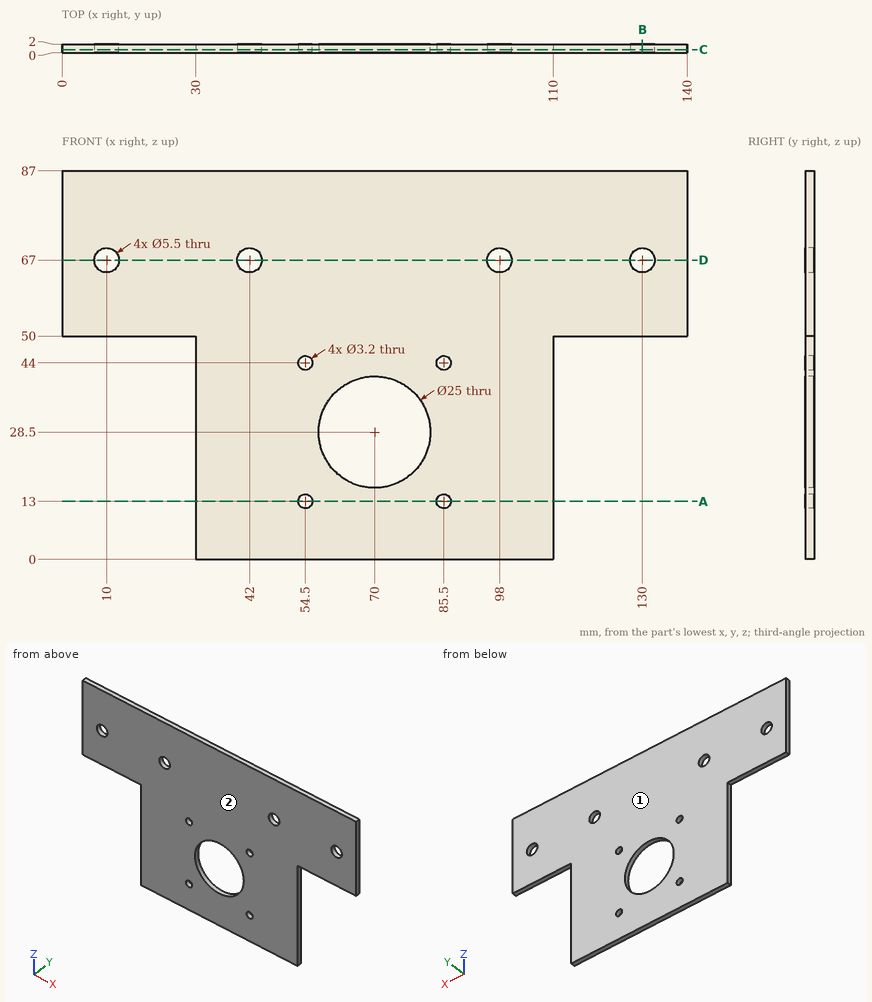
Could you check a few things on this drawing? It's one solid part, dimensions in mm from its lowest x, y, z. Coordinates: 2 decimals unless noted, no trailing zeros. Order: outer loops, then holes, each group sorted by start corner. A loop starts at its lowest first (then second) coordinate and runs counter-clockwise, first axis right, second up. Notation, with made-up numbers: M 5.25,37 L 44.25,37 A16 ccw 44.25,49 Z; hole C 42.25,20 d3. An arc over 180 degrees is marked long. Use one line per item in the form item = value. Start each with the question number.
1. We'd pull the mould along Y, two halves only. Please class the marked faces 1 and 2: +Y half, -Y half, draft (parallel to the pull), parting line (faces both ways), or undercut.
2. For pin 1 (12 mm diameter, centred on x = 124.5, z = 70.5, fed in from -Y); pin 2 (4.5 mm diameter, centred on x = 10, z = 67, fed in from -Y), each with a flat end and sliding along its axis, tell me the tip position at first contact or that it passes through.
3. Suppose I cut it at A-A on z = 13. Write out the boundary of the cut face in (x, y).
4. Please list where these lines run through material, in increasing order: line 1 (Z direction, x = 54.5, y = 1.4); line 2 (X direction, y = 1.55, z = 67); line 3 (Z direction, x = 130, y = 1.2).
5. Suppose I cut it at B-B on x = 130. Write out the boundary of the cut face in (y, z), then the cut area to 3 significant figures.
6. Suppose I cut it at C-C on y = 0.75. Count the separate pieces of the cut face and the enclosed holes in it, then the cut area to 3 significant figures.
7. Suppose I cut it at D-D on z = 67. Write out the boundary of the cut face in (x, y).
Geometry says:
q1.face_1 = +Y half
q1.face_2 = -Y half
q2.pin_1 = 0
q2.pin_2 = through
q3.outline = M 30,0 L 52.9,0 L 52.9,2 L 30,2 Z; M 56.1,0 L 83.9,0 L 83.9,2 L 56.1,2 Z; M 87.1,0 L 110,0 L 110,2 L 87.1,2 Z
q4.line_1 = 0 to 11.4, 14.6 to 42.4, 45.6 to 87
q4.line_2 = 0 to 7.25, 12.75 to 39.25, 44.75 to 95.25, 100.75 to 127.25, 132.75 to 140
q4.line_3 = 50 to 64.25, 69.75 to 87
q5.outline = M 0,50 L 2,50 L 2,64.25 L 0,64.25 Z; M 0,69.75 L 2,69.75 L 2,87 L 0,87 Z
q5.area = 63.0 mm^2
q6.separate_pieces = 1
q6.enclosed_holes = 9
q6.area = 8,560 mm^2
q7.outline = M 0,0 L 7.25,0 L 7.25,2 L 0,2 Z; M 12.75,0 L 39.25,0 L 39.25,2 L 12.75,2 Z; M 44.75,0 L 95.25,0 L 95.25,2 L 44.75,2 Z; M 100.75,0 L 127.25,0 L 127.25,2 L 100.75,2 Z; M 132.75,0 L 140,0 L 140,2 L 132.75,2 Z
